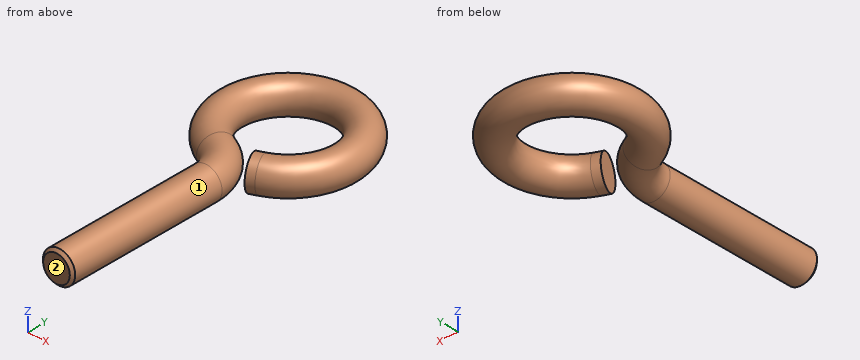
```python
from build123d import *

# Parameters (mm, degrees)
F1_R    = 2
F3_SIZE = 0.35


with BuildPart() as f2:
    # F2: sweep along a path in F0
    with BuildLine(Plane.XY) as f2_path:
        Line((0, 0), (0, 20))
        ThreePointArc((0, 20), (-0.8040266345, 22.7610739599), (-2.9647058824, 24.6588235294))
        ThreePointArc((-2.9647058824, 24.6588235294), (0.1135563879, 37.9990788642), (2.7574350901, 24.5659847899))
        Line((2.7574350901, 24.5659847899), (1.83829006, 24.1720654913))
    # F1 (on Front) → F2 (sweep)
    with BuildSketch(Plane.XZ):
        Circle(F1_R)
    sweep(path=f2_path.line)

    # F3
    f3_edges = [f2.edges().sort_by_distance(p)[0] for p in [
        (-2, 0, 0),
    ]]
    chamfer(f3_edges, length=F3_SIZE)


solid = f2.part
```
CAD build for the part. Positions are in the model's coordinates, mm. Face numbers are marked on the shaded views. A direction names the side the tool comes from. Round coordinates to 2 decimals unless told otherwise and drop trailing zeros. Order: outer loops, then holes, each group sorted by start corner. A loop starts at its lowest first (then second) coordinate and runs counter-clockwise, first axis right, second up.
Item 1: Saw through at A-A on z = 0. Write the cut outline in (x, y).
Item 2: Pin check, flat tips, straight feed: pin 1 (6 mm diameter, centred on x = 3.5, y = 18, fed in from -Z); pin 2 (2 mm diameter, centred on y = 33, z = 0.5, fed in from +X). Stop position of each tip, or through.
Item 3: Probe line 1 along X through (y, z) = (17, 0.15); line 2 along Y through (x, z) = (0.5, 0.65); line 3 along Y through (x, z) = (3.75, 1.4). List the from-to ranges inside material, lowest first.
Item 4: Saw through at B-B on y = 14. Write the cut outline in (x, z).
Item 5: Tool access for the marked faces 1 and 2: list every direction of +Z, -Z, +X, -X, +Y, -Y with a clear straight run to the whole face (end or side of a thin tool).
Reported:
1. outline: (-3.81, 22.85) arc R3.14 cw to (-2, 20) - (-2, 0.35) - (-1.65, 0) - (1.65, 0) - (2, 0.35) - (2, 20) arc R7.14 ccw to (-2.12, 26.47) arc R5 cw (long way) to (1.97, 26.4) - (1.05, 26.01) - (2.63, 22.33) - (3.55, 22.73) arc R9 ccw (long way) to start
2. pin 1: stops at z = -1.94
2. pin 2: stops at x = 8.93
3. line 1: x = -1.99 to 1.99
3. line 2: y = 0 to 24.2, 36.08 to 39.88
3. line 3: y = 23.45 to 26.88, 35.12 to 38.55
4. outline: circle Ø4 at (0, 0)
5. face 1: -Y
5. face 2: +Z, -Z, +X, -X, -Y
